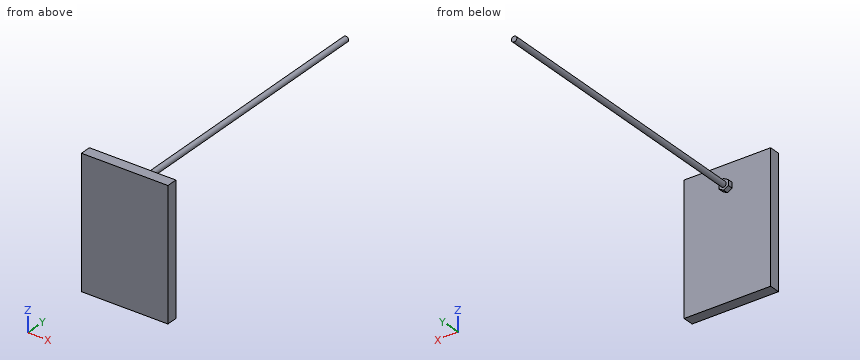
Autodesk Inventor part; units mm, degrees
ref_plane "YZ Plane" through (0, 0, 0) normal (1, 0, 0) x (0, 1, 0)
ref_plane "XZ Plane" through (0, 0, 0) normal (0, 1, 0) x (-1, 0, 0)
ref_plane "XY Plane" through (0, 0, 0) normal (0, 0, 1) x (1, 0, 0)
sketch "Sketch1" plane through (0, 0, 0) normal (0, 1, 0) x (-1, 0, 0)
  line L0 (0, 0) -> (203.2, 0)
  line L1 (203.2, 0) -> (203.2, -304.8)
  line L2 (203.2, -304.8) -> (0, -304.8)
  line L3 (0, -304.8) -> (0, 0)
  dimension "d0" = 203.2
  dimension "d1" = 304.8
extrude "Extrusion1" add sketch "Sketch1" along normal blind 25.4
sketch "Sketch2" plane through (0, 25.4, 0) normal (0, 1, 0) x (1, 0, 0)
  line L0 (-203.2, 0) -> (0, 0) construction
  line L1 (-101.6, 0) -> (-101.6, 50.8) construction
  line L2 (-101.6, 63.6316) -> (-90.4875, 57.2158)
  line L3 (-90.4875, 57.2158) -> (-90.4875, 44.3842)
  line L4 (-90.4875, 44.3842) -> (-101.6, 37.9684)
  line L5 (-101.6, 37.9684) -> (-112.7125, 44.3842)
  line L6 (-112.7125, 44.3842) -> (-112.7125, 57.2158)
  line L7 (-112.7125, 57.2158) -> (-101.6, 63.6316)
  dimension "d4" = 50.8
  dimension "d9" = 22.225
extrude "Extrusion2" add sketch "Sketch2" along normal blind 12.3031
sketch "Sketch3" plane through (0, 37.7031, 0) normal (0, 1, 0) x (1, 0, 0)
  line L0 (-112.7125, 57.2158) -> (-112.7125, 44.3842)
  line L1 (-112.7125, 44.3842) -> (-101.6, 37.9684)
  line L2 (-101.6, 37.9684) -> (-90.4875, 44.3842)
  line L3 (-90.4875, 44.3842) -> (-90.4875, 57.2158)
  line L4 (-90.4875, 57.2158) -> (-101.6, 63.6316)
  line L5 (-101.6, 63.6316) -> (-112.7125, 57.2158)
  line L6 (-101.6, 37.9684) -> (-112.7125, 44.3842) construction
  line L7 (-101.6, 63.6316) -> (-101.6, 37.9684) construction
  circle A0 centre (-101.6, 50.8) radius 6.35
  point P0 (0, 0)
  dimension "d8" = 12.7
extrude "Extrusion3" add sketch "Sketch3" along normal blind 670.56 contours A0
properties part number "Ring Stand"
Here's how the part is built. I have some questions about the finished solid (model axes, mm). Give positions to 0.01 mm unless a question says otherwise; leave off trailing zeros. Write each loop counter-clockwise with the first axis right and the second up, starting at its lowest first coordinate (ties: lowest second). Pieces come first, ordered by that corner, then holes. Notation, with made-up numbers: (67, 48.5) -> (115, 48.5) arc R16 ccw to (115, 59.5) -> close; hole circle Ø7 at (48.5, -7). An arc over 180 degrees is marked (long way). Use one line per item in the form item = value.
1) I'm going to push flat-ended pins straight in: pin 1 (3.5 mm diameter, centred on y = 29.5, z = -48, fed in from -X); pin 2 (3.5 mm diameter, centred on y = 32.5, z = -53, fed in from +X); pin 3 (10 mm diameter, centred on x = -132.5, z = -124.5, fed in from -Y); pin 4 (1.5 mm diameter, centred on x = -146.5, z = -183.5, fed in from +Y). Where does each tip first touch, or does it pass through?
Verdict:
pin_1 = -112.71
pin_2 = -90.49
pin_3 = 0
pin_4 = 25.4
2) Suppose I cut it at A-A (z = -125.5). Please give me the cut outline in (x, y), and give its area (3 significant figures).
Verdict:
outline = (-203.2, 0) -> (0, 0) -> (0, 25.4) -> (-203.2, 25.4) -> close
area = 5,160 mm2
3) Suppose I cut it at C-C (y = 590.5). Please give me the cut outline in (x, z).
Verdict:
outline = circle Ø12.7 at (-101.6, -50.8)
4) If I drill on L1, parallel to Y at x = -25.5, z = -111.5; L2, parallel to X at y = 486.5, z = -51.5; L3, parallel to Z at x = -99.5, y = 641, over which ranges is the centre line in solid material (lowest first)? Write a range as [from, to].
Verdict:
L1 = [0, 25.4]
L2 = [-107.91, -95.29]
L3 = [-56.79, -44.81]
5) Suppose I cut it at B-B (x = -157.5). Please give me the cut outline in (y, z), and give its area (3 significant figures).
Verdict:
outline = (0, -304.8) -> (25.4, -304.8) -> (25.4, 0) -> (0, 0) -> close
area = 7,740 mm2
